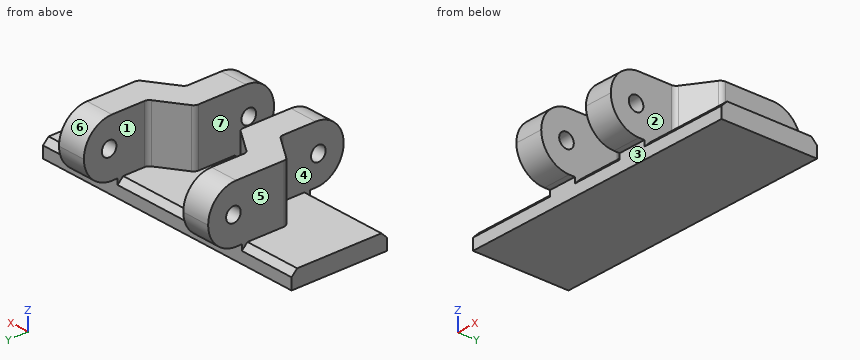
```python
from build123d import *

# Parameters (mm, degrees)
ESQUISSE1_W                     = 50
ESQUISSE1_H                     = 17
BOSS_EXTRU_1_DEPTH              = 3
BOSS_EXTRU_2_DEPTH              = 10
CONG_1_R                        = 5
CONG_2_R                        = 1
CHANFREIN1_SIZE                 = 1
DIAM_TRE_DU_PER_AGE_2_6_2_6_1_D = 2.6


with BuildPart() as part:
    # Esquisse1 → Boss.-Extru.1 (new body)
    with BuildSketch(Plane.XY):
        Rectangle(ESQUISSE1_W, ESQUISSE1_H)
    extrude(amount=BOSS_EXTRU_1_DEPTH)

    # Esquisse2 → Boss.-Extru.2 (add)
    with BuildSketch(Plane.XY.offset(3)):
        Polygon((-15, 14.5), (-15, 0.5), (-9.5, -3.173254132), (-9.5, -14.5), (-4.5, -14.5), (-4.5, -0.5), (-10, 3.173254132), (-10, 14.5), align=None)
        Polygon((10, 14.5), (15, 14.5), (15, 0.5), (9.5, -3.173254132), (9.5, -14.5), (4.5, -14.5), (4.5, -0.5), (10, 3.173254132), align=None)
    extrude(amount=BOSS_EXTRU_2_DEPTH)

    # Congé1
    cong_1_edges = [part.edges().sort_by_distance(p)[0] for p in [
        (7, -14.5, 13),
        (7, -14.5, 3),
        (-7, -14.5, 3),
        (-7, -14.5, 13),
        (-12.5, 14.5, 13),
        (12.5, 14.5, 13),
        (12.5, 14.5, 3),
        (-12.5, 14.5, 3),
    ]]
    fillet(cong_1_edges, radius=CONG_1_R - 0.0001)  # a hair under: the kernel refuses the full size

    # Congé2
    cong_2_edges = [part.edges().sort_by_distance(p)[0] for p in [
        (-15, 0.5, 8),
        (-9.5, -3.173254132, 8),
        (-4.5, -0.5, 8),
        (-10, 3.173254132, 8),
        (10, 3.173254132, 8),
        (4.5, -0.5, 8),
        (9.5, -3.173254132, 8),
        (15, 0.5, 8),
    ]]
    fillet(cong_2_edges, radius=CONG_2_R)

    # Chanfrein1
    chanfrein1_edges = [part.edges().sort_by_distance(p)[0] for p in [
        (-17.25, -8.5, 3),
        (-20, 8.5, 3),
        (0, -8.5, 3),
        (17.25, -8.5, 3),
        (0, 8.5, 3),
        (20, 8.5, 3),
    ]]
    chamfer(chanfrein1_edges, length=CHANFREIN1_SIZE)

    # Diamètre du perçage Ø2.6 (2.6)1 (through all)
    with Locations(Plane(origin=(15, 0, 0), x_dir=(0, 0, -1), z_dir=(1, 0, 0))):
        with Locations((-8, -10), (-8, 10)):
            Hole(DIAM_TRE_DU_PER_AGE_2_6_2_6_1_D / 2)


solid = part.part
```
Geometry: final body of the model. Coordinates: model frame, mm. Face numbers are marked on the shaded views. A direction names the side the tool comes from. Give positions to 0.01 mm unless a question says otherwise; leave off trailing zeros. Write each loop counter-clockwise with the first axis right and the second up, starting at its lowest first coordinate (ties: lowest second). Pieces come first, ordered by that corner, then holes.
1. Pin query (flat end, axial travel): P1, Ø1.6, axis at y = 10, z = 8, coming from the -X side; P2, Ø4, axis at x = 14.5, z = 10, coming from the +Y side; P3, Ø5, axis at x = -0.5, y = 0.5, coming from the +Z side; P4, Ø2.5, axis at x = -7.5, z = 1.5, coming from the +Y side. Return the tip coordinate at first contact, or that it passes through.
2. Section query C-C, the plane y = 5.5. Return loops of the section in (x, z), then the cut area to 3 significant figures.
3. Reachability of the marked faces 1, 2, 3 and 4 from +Z, -Z, +X, -X, +Y, -Y: full face, straight path, thin tool, end or side. Return the list, or none.
4. Section query B-B, the plane z = 11. Return loops of the section in (x, y), then the cut area to 3 significant figures.
5. Section query D-D, the plane x = -0.5. Return loops of the section in (y, z), then the cut area to 3 significant figures.
6. Section query A-A, the plane y = -10. Return loops of the section in (x, z).
7. Line query: probe 1 along X at (y, z) = (-4.25, 12.75); probe 2 along X at (y, z) = (9.5, 12); probe 3 along Y at (x, z) = (-2.5, 2). Output: solid intervals per line, ascending.
8. Draft query along X for the marked faces 5, 6 and 7. Return one class per face: released by +X, released by -X, zero draft, split by the parting line, or undercut.
Computed:
1. P1: passes through
1. P2: stops at y = 14.5
1. P3: stops at z = 3
1. P4: stops at y = 8.5
2. outline: (-25, 0) - (25, 0) - (25, 3) - (15, 3) - (15, 13) - (10, 13) - (10, 3) - (-10, 3) - (-10, 13) - (-15, 13) - (-15, 3) - (-25, 3) - close
2. area: 250 mm2
3. face 1: +Z, +Y
3. face 2: +Z, +X, -Y
3. face 3: -Z, +X, -X, -Y
3. face 4: +Z, -X, -Y
4. outline: (-15, 1.03) arc R1 ccw to (-14.56, 0.2) - (-9.94, -2.88) arc R1 cw to (-9.5, -3.71) - (-9.5, -13.5) - (-4.5, -13.5) - (-4.5, -1.03) arc R1 ccw to (-4.94, -0.2) - (-9.56, 2.88) arc R1 cw to (-10, 3.71) - (-10, 13.5) - (-15, 13.5) - close; (4.5, -13.5) - (9.5, -13.5) - (9.5, -3.71) arc R1 cw to (9.94, -2.88) - (14.56, 0.2) arc R1 ccw to (15, 1.03) - (15, 13.5) - (10, 13.5) - (10, 3.71) arc R1 cw to (9.56, 2.88) - (4.94, -0.2) arc R1 ccw to (4.5, -1.03) - close
4. area: 299 mm2
5. outline: (-8.5, 0) - (8.5, 0) - (8.5, 2) - (7.5, 3) - (-7.5, 3) - (-8.5, 2) - close
5. area: 50.0 mm2
6. outline: (-9.5, 3.03) - (-4.5, 3.03) - (-4.5, 6.7) - (-9.5, 6.7) - close; (-9.5, 9.3) - (-4.5, 9.3) - (-4.5, 12.97) - (-9.5, 12.97) - close; (4.5, 3.03) - (9.5, 3.03) - (9.5, 6.7) - (4.5, 6.7) - close; (4.5, 9.3) - (9.5, 9.3) - (9.5, 12.97) - (4.5, 12.97) - close
7. probe 1: x = -9.5 to -4.5, 4.5 to 9.5
7. probe 2: x = -15 to -10, 10 to 15
7. probe 3: y = -8.5 to 8.5
8. face 5: released by -X
8. face 6: zero draft
8. face 7: undercut
